```python
from build123d import *

# Parameters (mm, degrees)
COPYSKETCH018_W             = 6.8
COPYSKETCH018_H             = 3.7
CYLINDER069_R               = 3.1
CYLINDER069_DEPTH           = 44
CYLINDER069_ROLL_ANGLE      = -89.999777
CYLINDER069_PITCH_ANGLE     = -2.5e-05
CYLINDER069_PLACEMENT_ANGLE = 7.5e-05
SKETCH022_R                 = 3.1
PAD022_DEPTH                = 16


with BuildPart() as obj1:
    # CopySketch018 → Revolution004 (revolve)
    with BuildSketch(Plane.YZ):
        with Locations((-5.899207, -4.35)):
            Rectangle(COPYSKETCH018_W, COPYSKETCH018_H)
    revolve(axis=Axis((0, 0, 0), (0, 1, 0)))


with BuildPart() as obj1_1:
    # Body032 placement: moved
    add(obj1.part.moved(Location((0, -4.4, 0))))


with BuildPart() as bohrung_durch_innen:
    # Cylinder069 → Cylinder069 (new body)
    with BuildSketch(Plane.XY):
        Circle(CYLINDER069_R)
    extrude(amount=CYLINDER069_DEPTH)


with BuildPart() as bohrung_durch_innen_1:
    # Cylinder069 roll: moved
    add(bohrung_durch_innen.part.rotate(Axis((0, 0, 0), (1, 0, 0)), CYLINDER069_ROLL_ANGLE))


with BuildPart() as bohrung_durch_innen_2:
    # Cylinder069 pitch: moved
    add(bohrung_durch_innen_1.part.rotate(Axis((0, 0, 0), (0, 1, 0)), CYLINDER069_PITCH_ANGLE))


with BuildPart() as bohrung_durch_innen_3:
    # Cylinder069 placement: moved
    add(bohrung_durch_innen_2.part.moved(Location((-0.041441, -44.040796, -8.4e-05))).rotate(Axis((-0.041441, -44.040796, -8.4e-05), (0, 0, 1)), CYLINDER069_PLACEMENT_ANGLE))


with BuildPart() as obj2:
    # Sketch023 → Revolution (revolve)
    with BuildSketch(Plane.XZ):
        Polygon((-12.204835, 0), (-12.204835, -4.1), (-5, -4.1), (-5, -2.6), (5, -2.6), (5, -4.1), (12.102632, -4.1), (12.102632, 0), align=None)
    revolve(axis=Axis((0, 0, 0), (1, 0, 0)))


with BuildPart() as obj2_1:
    # Body033 placement: moved
    add(obj2.part.moved(Location((0, -17.1, -12))))


with BuildPart() as cut064:
    # Sketch022 → Pad022 (new body)
    with BuildSketch(Plane.XZ):
        with BuildLine():
            Line((-9, 7), (-6.4, 9.6))
            Line((-6.4, 9.6), (6.4, 9.6))
            Line((6.4, 9.6), (9, 7))
            Line((9, 7), (9, -19))
            ThreePointArc((-9, -19), (0, -21.023796), (9, -19))
            Line((-9, -19), (-9, 7))
        make_face()
        Circle(SKETCH022_R, mode=Mode.SUBTRACT)
    extrude(amount=PAD022_DEPTH)


with BuildPart() as cut064_1:
    # Body031 placement: moved
    add(cut064.part.moved(Location((0, -8.9, 0))))

    # Cut062: cut obj2
    add(obj2_1.part, mode=Mode.SUBTRACT)

    # Cut063: cut bohrung-durch-innen
    add(bohrung_durch_innen_3.part, mode=Mode.SUBTRACT)

    # Cut064: cut obj1
    add(obj1_1.part, mode=Mode.SUBTRACT)


solid = cut064_1.part
```
Geometry: final body of the model. Coordinates: model frame, mm. A direction names the side the tool comes from. Round coordinates to 2 decimals unless told otherwise and drop trailing zeros. Order: outer loops, then holes, each group sorted by start corner. A loop starts at its lowest first (then second) coordinate and runs counter-clockwise, first axis right, second up. Notation, with made-up numbers: (9.5, -37) - (61.5, -37) arc R25 ccw to (61.5, -4) - close; hole circle Ø10 at (74, -33). An arc over 180 degrees is marked (long way). Write item = value, one per line. Start each with the question number.
Q1. Pull-direction query (Z, two-part tool) for faces 1 (the flat face through (5, -17, -9)), 2 (the flat face through (-8, -17, 8)), 3 (the flat face through (9, -17, -6)); classes: +Z half, -Z half, draft (parallel to the pull), parting line (faces both ways), or undercut.
Q2. Cut plane B-B on x = 2.5. Return the cut outline in (y, z).
Q3. Cut plane D-D on x = -4.5. Return the cut outline in (y, z).
Q4. Ray query, line 1 (Y direction, x = -7.5, z = -12); line 2 (Y direction, x = 0.5, z = -12); line 3 (Z direction, x = -1.75, y = -15.5). Return the intervals inside material, ascending. Write a range as from..to.
Q5. Pin query (flat end, axial travel): pin 1 (2.5 mm diameter, centred on y = -17.5, z = -13.5, fed in from +X); pin 2 (4 mm diameter, centred on y = -17, z = -14, fed in from -X); pin 3 (6 mm diameter, centred on x = 7, y = -19.5, fed in from -Z). Return the tip coordinate at first contact, or that it passes through.
Q6. Cut plane A-A on z = -12. Return the cut outline in (x, y).
Q7. Cut plane C-C on y = -17.1. Give the number of separate pieces and of enclosed holes in the cut face, and give its area (3 significant figures).
Q8. Access query for faces 4 (the cylindrical face through (-1.9, -11.3, -5.9)), 5 (the cylindrical face through (7.028, -14.329, -8.978)), 6 (the flat face through (-5, -17, -15)). Directions: +Z, -Z, +X, -X, +Y, -Y. A direction counts if a zero-diameter tool reaches every point of the face in a straight line with its end or side. Return the directions, or none.
Outcome:
q1.face_1 = undercut
q1.face_2 = +Z half
q1.face_3 = draft
q2.outline = (-24.9, -20.87) - (-8.9, -20.87) - (-8.9, -5.67) - (-13.7, -5.67) - (-13.7, -1.83) - (-24.9, -1.83) - close; (-24.9, 1.83) - (-13.7, 1.83) - (-13.7, 5.67) - (-8.9, 5.67) - (-8.9, 9.6) - (-24.9, 9.6) - close; hole circle Ø5.2 at (-17.1, -12)
q3.outline = (-24.9, -20.54) - (-8.9, -20.54) - (-8.9, -4.26) - (-13.7, -4.26) - (-13.7, 4.26) - (-8.9, 4.26) - (-8.9, 9.6) - (-24.9, 9.6) - close; hole circle Ø5.2 at (-17.1, -12)
q4.line_1 = -24.9..-21.2, -13..-8.9
q4.line_2 = -24.9..-19.7, -14.5..-8.9
q4.line_3 = -20.95..-14.05, -9.95..-2.59, 2.59..9.6
q5.pin_1 = 5
q5.pin_2 = -5
q5.pin_3 = -20.64
q6.outline = (-9, -24.9) - (9, -24.9) - (9, -21.2) - (5, -21.2) - (5, -19.7) - (-5, -19.7) - (-5, -21.2) - (-9, -21.2) - close; (-9, -13) - (-5, -13) - (-5, -14.5) - (5, -14.5) - (5, -13) - (9, -13) - (9, -8.9) - (-9, -8.9) - close
q7.separate_pieces = 2
q7.enclosed_holes = 1
q7.area = 385 mm^2
q8.face_4 = +Y
q8.face_5 = +X
q8.face_6 = -X
